Autodesk Inventor part; units mm, degrees
ref_plane "YZ Plane" through (0, 0, 0) normal (1, 0, 0) x (0, 1, 0)
ref_plane "XZ Plane" through (0, 0, 0) normal (0, 1, 0) x (-1, 0, 0)
ref_plane "XY Plane" through (0, 0, 0) normal (0, 0, 1) x (1, 0, 0)
sketch "Skizze1" plane through (0, 0, 0) normal (0, 0, 1) x (1, 0, 0)
  line L0 (-259, 0) -> (259, 0)
  line L1 (0, -289.7487) -> (0, 264.1248)
  circle A0 centre (0, 0) radius 185
  line L2 (-40, -180.6239) -> (40, -180.6239)
  line L3 (-40, -180.6239) -> (-40, -210.6239)
  line L4 (-40, -210.6239) -> (40, -210.6239)
  line L5 (40, -210.6239) -> (40, -180.6239)
  point P0 (0, -180.6239)
  dimension "d0" = 370
  dimension "d1" = 80
  dimension "d2" = 40
  dimension "d3" = 0
  dimension "d4" = 30
extrude "Extrusion1" add sketch "Skizze1" along normal blind 30 contours A0 L1 L4 L3 | A0 L5 L4 L1
sketch "Skizze2" plane through (-40, -210.6239, 0) normal (0, -1, 0) x (1, 0, 0)
  point P0 (40, 0)
sketch "Skizze3" plane through (-40, -210.6239, 0) normal (0, -1, 0) x (1, 0, 0)
  line L0 (2.5, 2.5) -> (77.5, 2.5)
  line L1 (77.5, 2.5) -> (77.5, 27.5)
  line L2 (77.5, 27.5) -> (2.5, 27.5)
  line L3 (2.5, 27.5) -> (2.5, 2.5)
  line L4 (0, 0) -> (0, 30)
  line L5 (0, 0) -> (80, 0)
  line L6 (0, 30) -> (80, 30)
  line L7 (80, 0) -> (80, 30)
  point P0 (40, 0)
  dimension "d7" = 2.5
  dimension "d8" = 2.5
  dimension "d9" = 2.5
  dimension "d10" = 2.5
extrude "Extrusion2" cut sketch "Skizze3" against normal blind 30 contours L3 L2 L1 L0
sketch "Skizze4" plane through (-40, -210.6239, 0) normal (0, -1, 0) x (1, 0, 0)
  line L0 (2.5, 27.5) -> (2.5, 2.5)
  line L1 (77.5, 27.5) -> (77.5, 2.5)
  line L2 (2.5, 2.5) -> (77.5, 2.5)
  line L3 (77.5, 2.5) -> (77.5, 27.5)
  line L4 (77.5, 27.5) -> (2.5, 27.5)
  line L5 (2.5, 27.5) -> (2.5, 2.5)
  point P0 (40, 0)
extrude "Extrusion3" add sketch "Skizze4" against normal blind 2.5
sketch "Skizze5" plane through (-40, -210.6239, 0) normal (0, -1, 0) x (1, 0, 0)
  line L0 (0, 0) -> (0, 30)
  point P0 (40, 0)
  point P1 (40, 15)
  dimension "d15" = 40
  dimension "d16" = 15
hole "Bohrung1" at (0, -210.6239, 15) direction (0, 1, 0) diameter 9.3762 end through all
properties part number "WasserAblauf1"
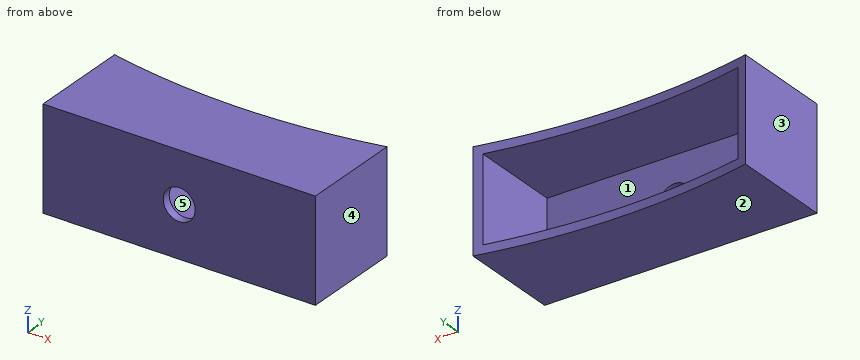
Geometry check sheet. Reference: the model listing, model coordinates, mm. Face numbers are marked on the shaded views. A direction names the side the tool comes from. Give positions to 0.01 mm unless a question says otherwise; leave off trailing zeros. Loops run counter-clockwise (first coordinate to the right, second up) from the corner with the lowest first, then second, coordinate; pieces in that order, holes last. Notation, with made-up numbers: (-23, 27.25) - (27, 27.25) arc R22 ccw to (27, 51.25) - close; hole circle Ø6 at (-25, 45). An arc over 180 degrees is marked (long way). Use CSV: the item, a comma, the result in double quotes. Start each with the question number.
Q1. Scan lines: probe 1 along X at (y, z) = (-202.75, 24); probe 2 along X at (y, z) = (-210.05, 15); probe 3 along Z at (x, y) = (0, -209.8). Record each from-to range of solid material in increasing order. Write a range as from..to.
Q2. Release check for a two-part mould opening along Z. For the marked faces 1, 2 and 3 record: +Z half, -Z half, draft (parallel to the pull), parting line (faces both ways), or undercut.
Q3. Go/stop test with flat-tipped pins: pin 1 Ø6 at (x, z) = (-23.5, 27) entering from +Y; pin 2 Ø11 at (x, z) = (0, 15) entering from +Y. Record where each tip stops, or that it passes through.
Q4. Section check B-B, the plane x = 0. Record the cut outline in (y, z).
Q5. Section check C-C, the plane y = -182.5. Record the cut outline in (x, z).
Q6. Section check D-D, the plane z = 15. Record the cut outline in (x, y), and give its area (3 significant figures).
Q7. Section check A-A, the plane y = -193.75. Record the cut outline in (x, z), and give its area (3 significant figures).
Q8. Access from +Z, -Z, +X, -X, +Y, -Y to the whole of each face (thin tool, end or side, straight path). Record for the marked faces 4 and 5.
Findings below:
1,probe 1,"x = -40..-37.5, 37.5..40"
1,probe 2,"x = -40..-4.69, 4.69..40"
1,probe 3,"z = 0..10.31, 19.69..30"
2,face 1,"undercut"
2,face 2,"-Z half"
2,face 3,"draft"
3,pin 1,"stops at y = -183.1"
3,pin 2,"stops at y = -208.12"
4,outline,"(-210.62, 0) - (-185, 0) - (-185, 2.5) - (-208.12, 2.5) - (-208.12, 10.31) - (-210.62, 10.31) - close; (-210.62, 19.69) - (-208.12, 19.69) - (-208.12, 27.5) - (-185, 27.5) - (-185, 30) - (-210.62, 30) - close"
5,outline,"(-40, 0) - (-30.31, 0) - (-30.31, 2.5) - (-37.5, 2.5) - (-37.5, 27.5) - (-30.31, 27.5) - (-30.31, 30) - (-40, 30) - close; (30.31, 0) - (40, 0) - (40, 30) - (30.31, 30) - (30.31, 27.5) - (37.5, 27.5) - (37.5, 2.5) - (30.31, 2.5) - close"
6,outline,"(-40, -210.62) - (-4.69, -210.62) - (-4.69, -208.12) - (-37.5, -208.12) - (-37.5, -181.16) arc R185 cw to (-40, -180.62) - close; (4.69, -210.62) - (40, -210.62) - (40, -180.62) arc R185 cw to (37.5, -181.16) - (37.5, -208.12) - (4.69, -208.12) - close"
6,area,"313 mm^2"
7,outline,"(-40, 0) - (40, 0) - (40, 30) - (-40, 30) - close; hole (-37.5, 2.5) - (37.5, 2.5) - (37.5, 27.5) - (-37.5, 27.5) - close"
7,area,"525 mm^2"
8,face 4,"+Z, -Z, +X, +Y, -Y"
8,face 5,"+Y"
